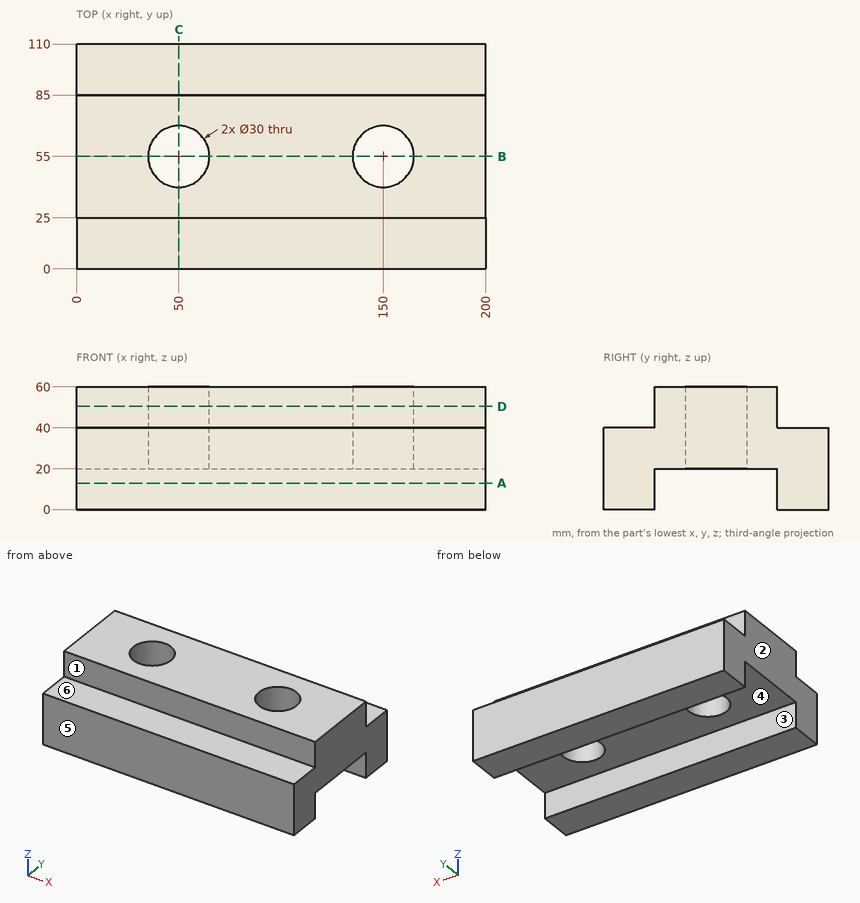
The drawing under review shows one solid part. Ordinate dimensions are in mm from its lowest x, y, z. A direction names the side the tool comes from. Round coordinates to 2 decimals unless told otherwise and drop trailing zeros. Loops run counter-clockwise (first coordinate to the right, second up) from the corner with the lowest first, then second, coordinate; pieces in that order, holes last. Notation, with made-up numbers: (-10.5, 9.5) - (26.5, 9.5) arc R31 ccw to (26.5, 37.5) - close; hole circle Ø10 at (-23.75, -26). An arc over 180 degrees is marked (long way). One line per item, written item: value. Start each with the question number.
1) For the marked faces 4, 5 and 6, list the 3-axis set-ups (+Z, -Z, +X, -X, +Y, -Y) from which the entire face can be reached by the end or side of a thin tool; tool diameter is ignored.
2) Consider section A-A on z = 13. Give the boundary of the cut face in (x, y).
3) Consider section C-C on x = 50. Give the boundary of the cut face in (y, z).
4) Insertion check: pin 1 Ø20 at (x, y) = (147.5, 100.5) entering from +Z; pin 2 Ø6 at (x, z) = (54, 47) entering from -Y; pin 3 Ø5 at (x, y) = (38, 79) entering from -Z. Each pin has a flat end and moves straight along its axis. Give the tip position at first contact, or say it passes through.
5) Consider section B-B on y = 55. Give the boundary of the cut face in (x, z).
6) Draft analysis for pull direction Y (two halves, no side actions). For the marked faces 1, 2 and 3, state which applies: +Y half, -Y half, draft (parallel to the pull), parting line (faces both ways), or undercut.
7) To check wall thickness, follow L1, parallel to Y at x = 50, z = 44; L2, parallel to Y at x = 150, z = 36; L3, parallel to X at y = 65, z = 52.5. State the ranges of each line that lie inside material, in increasing order. Write a range as from..to.
8) Consider section D-D on z = 50.5. Give the boundary of the cut face in (x, y).
Reported:
1. face 4: -Z, +X, -X
1. face 5: +Z, -Z, +X, -X, -Y
1. face 6: +Z, +X, -X, -Y
2. outline: (0, 0) - (200, 0) - (200, 25) - (0, 25) - close; (0, 85) - (200, 85) - (200, 110) - (0, 110) - close
3. outline: (0, 0) - (25, 0) - (25, 20) - (40, 20) - (40, 60) - (25, 60) - (25, 40) - (0, 40) - close; (70, 20) - (85, 20) - (85, 0) - (110, 0) - (110, 40) - (85, 40) - (85, 60) - (70, 60) - close
4. pin 1: stops at z = 40
4. pin 2: stops at y = 25
4. pin 3: stops at z = 20
5. outline: (0, 20) - (35, 20) - (35, 60) - (0, 60) - close; (65, 20) - (135, 20) - (135, 60) - (65, 60) - close; (165, 20) - (200, 20) - (200, 60) - (165, 60) - close
6. face 1: -Y half
6. face 2: draft
6. face 3: undercut
7. L1: y = 25..40, 70..85
7. L2: y = 0..40, 70..110
7. L3: x = 0..38.82, 61.18..138.82, 161.18..200
8. outline: (0, 25) - (200, 25) - (200, 85) - (0, 85) - close; hole circle Ø30 at (50, 55); hole circle Ø30 at (150, 55)
